Geometry check sheet. Reference: the model listing, model coordinates, mm. Give positions to 0.01 mm unless a question says otherwise; leave off trailing zeros. Order: outer loops, then holes, each group sorted by start corner. A loop starts at its lowest first (then second) coordinate and runs counter-clockwise, first axis right, second up. Notation, with made-up numbers: M -5,-9 L 38,-9 A19 ccw 38,27 Z; hole C 55.5,78 d11. An arc over 180 degrees is marked long. Answer as a JSON object with one key per item and string values. Group by question number.
from build123d import *

# Parameters (mm, degrees)
SKETCH_1_W          = 40
SKETCH_1_H          = 20
SKETCH_1_R          = 7
EXTRUDE_1_DEPTH     = 20
SKETCH_2_R          = 5
CUT_EXTRUDE_1_DEPTH = 41


with BuildPart() as part:
    # 草图1 → 凸台-拉伸1 (new body)
    with BuildSketch(Plane.XY):
        Rectangle(SKETCH_1_W, SKETCH_1_H)
        Circle(SKETCH_1_R, mode=Mode.SUBTRACT)
    extrude(amount=EXTRUDE_1_DEPTH)

    # 草图2 → 切除-拉伸1 (cut, through all)
    with BuildSketch(Plane.ZY.offset(20)):
        with Locations((10, 0)):
            Circle(SKETCH_2_R)
    extrude(amount=-CUT_EXTRUDE_1_DEPTH, mode=Mode.SUBTRACT)


solid = part.part
1. Thickness scan on line 1 along Y through (x, z) = (10, 10); line 2 along Y through (x, z) = (0, 16.25); line 3 along Z through (x, y) = (-14.25, 0). Record the ranges inside material, lowest first. Write a range as [from, to].
2. Cross-section at A-A (y = 0). Record the cut outline in (x, z), and give its area (3 significant figures).
3. Cross-section at B-B (z = 10). Record the cut outline in (x, y), and give its area (3 significant figures).
4. Cross-section at D-D (x = -6). Record the cut outline in (y, z), and give its area (3 significant figures).
5. Cross-section at C-C (x = -16). Record the cut outline in (y, z), and give its area (3 significant figures).
6. Release check for a two-part mould opening along Y. For faces 1 (the flat face through (20, -2, 5)), 2 (the cylindrical face through (12.34, 1.5, 14.77)), 3 (the flat face through (0, 10, 10)) record: released by +Y, released by -Y, zero draft, split by the parting line, or undercut.
Report:
{
 "1": {"line 1": "y = [-10, -5], [5, 10]", "line 2": "y = [-10, -7], [7, 10]", "line 3": "z = [0, 5], [15, 20]"},
 "2": {"outline": "M -20,0 L -7,0 L -7,5 L -20,5 Z; M -20,15 L -7,15 L -7,20 L -20,20 Z; M 7,0 L 20,0 L 20,5 L 7,5 Z; M 7,15 L 20,15 L 20,20 L 7,20 Z", "area": "260 mm2"},
 "3": {"outline": "M -20,-10 L 20,-10 L 20,-5 L 4.9,-5 A7 cw -4.9,-5 L -20,-5 Z; M -20,5 L -4.9,5 A7 cw 4.9,5 L 20,5 L 20,10 L -20,10 Z", "area": "373 mm2"},
 "4": {"outline": "M -10,0 L -3.61,0 L -3.61,6.54 A5 cw -3.61,13.46 L -3.61,20 L -10,20 Z; M 3.61,0 L 10,0 L 10,20 L 3.61,20 L 3.61,13.46 A5 cw 3.61,6.54 Z", "area": "242 mm2"},
 "5": {"outline": "M -10,0 L 10,0 L 10,20 L -10,20 Z; hole C 0,10 d10", "area": "321 mm2"},
 "6": {"face 1": "zero draft", "face 2": "undercut", "face 3": "released by +Y"}
}
